Here's how the part is built. I have some questions about the finished solid (model axes, mm). A direction names the side the tool comes from. Coordinates: 2 decimals unless noted, no trailing zeros. Answer as CSV lines item,"result". Start each with the question number.
Item 1: I'm going to push flat-ended pins straight in: pin 1 (1.5 mm diameter, centred on x = -1, z = 0, fed in from -Y); pin 2 (1.5 mm diameter, centred on x = 7.5, y = -1.5, fed in from -Z); pin 3 (1.6 mm diameter, centred on x = 11, z = -0.5, fed in from +Y). Where does each tip first touch, or does it pass through?
Item 2: I need wall thicknesses on line 1 (Y direction, x = -3.5, z = 0); line 2 (Y direction, x = -3.5, z = -0.75); line 3 (X direction, y = 0.45, z = -0.4). Which ranges of each line are inside material? Lowest first, please.
Item 3: On a 3-axis mill with a long thin cutter (end or side, diameter ignored), from which of +Z, -Z, +X, -X, +Y, -Y can I reach the whole of each face in a straight line? I mean faces 1 (the face through (22.633, -0.407, -0.022)), 2 (the face through (9.9, 1.6, 0)), 3 (the face through (11.8, -1.6, 0)). Say none if no direction works.
from build123d import *

# Parameters (mm, degrees)
CONECUT_DEPTH      = 2.59999885
CONECUT_DEPTH_BACK = 2.59999885


with BuildPart() as part:
    # Body: sweep along a path in 草图2
    with BuildLine(Plane.XY) as body_path:
        Line((20, 1.6), (0, 1.6))
        ThreePointArc((0, 1.6), (-0.857074534, 1.7540301), (-1.606886657, 2.196843615))
        ThreePointArc((-1.606886657, 2.196843615), (-6.4, 0), (-1.606886657, -2.196843615))
        ThreePointArc((-1.606886657, -2.196843615), (-0.857074534, -1.7540301), (0, -1.6))
        Line((0, -1.6), (23.2, -1.6))
    # 草图1 → Body (sweep)
    with BuildSketch(Plane(origin=(20, 0, 0), x_dir=(0, 0, -1), z_dir=(1, 0, 0))):
        with BuildLine():
            Line((-1.59999875, 0.002), (1.59999875, 0.002))
            ThreePointArc((1.59999875, 0.002), (0, 1.6), (-1.59999875, 0.002))
        make_face()
    sweep(path=body_path.line)

    # 草图3 → ConeCut (cut, two sides)
    with BuildSketch(Plane.XY) as conecut_sk:
        Polygon((20, 0.801), (18.853141685, 1.61), (23.21, 1.61), (23.21, -1.61), (22.053141685, -1.61), (23.2, -0.801), (22.047540024, 0), (18.847540024, 0), align=None)
    extrude(amount=CONECUT_DEPTH, mode=Mode.SUBTRACT)
    extrude(conecut_sk.sketch, amount=-CONECUT_DEPTH_BACK, mode=Mode.SUBTRACT)


solid = part.part
Responses:
1,pin 1,"stops at y = -2.31"
1,pin 2,"stops at z = -1.41"
1,pin 3,"stops at y = 1.6"
2,line 1,"y = -2.9 to -1.3, 1.3 to 2.9"
2,line 2,"y = -2.71 to -1.3, 1.3 to 2.71"
2,line 3,"x = -6.31 to -4.72, -1.85 to 19.49"
3,face 1,"+Z, -Z, +X, +Y"
3,face 2,"+X, +Y"
3,face 3,"+X, -Y"
